Here's how the part is built. I have some questions about the finished solid (model axes, mm). A direction names the side the tool comes from. Round coordinates to 2 decimals unless told otherwise and drop trailing zeros. Write each loop counter-clockwise with the first axis right and the second up, starting at its lowest first coordinate (ties: lowest second). Pieces come first, ordered by that corner, then holes. Notation, with made-up numbers: M 71,8 L 85,8 A32 ccw 85,37 Z; hole C 14,15 d11. An arc over 180 degrees is marked long. Use one line per item in the form item = value. Start each with the question number.
Q1. I want a section at C-C on y = -13. List the corners of the cut face in (x, z) for me, and give its area (3 significant figures).
Q2. I want a section at B-B on y = 17.5. List the corners of the cut face in (x, z) for me.
Q3. I need wall thicknesses on line 1 along X through (y, z) = (-31, 13.25); line 2 along X through (y, z) = (-0.5, 5); line 3 along X through (y, z) = (-28, 2.75). Which ranges of each line are inside material? Lowest first, please. Write a range as from..to.
Q4. I want a section at A-A on z = 7.5. List the corners of the cut face in (x, y) for me, and give its area (3 significant figures).
Q5. We'd pull the mould along X, two halves only. Please class faces 4 (the face through (-19.46, -48.22, 7.4)), 5 (the face through (19.076, -48.375, 7.395)), 6 (the face through (0, 31, 8)): +X half, -X half, draft (parallel to the pull), parting line (faces both ways), or undercut.
Q6. I want a section at D-D on x = 43.5. List the corners of the cut face in (y, z) for me, and give its area (3 significant figures).
Q7. For faces 1 (the face through (5, -46, 8)), 2 (the face through (-46.99, 0.05, 6.25)), 3 (the face through (11, 1, 15)), which set-ups out of +Z, -Z, +X, -X, +Y, -Y let a thin tool reach every point of the face, with its end or its side?
Q8. I'm going to push flat-ended pins straight in: pin 1 Ø5 at (y, z) = (-18, 9.5) entering from +X; pin 2 Ø6 at (x, z) = (40.5, 13) entering from -Y; pin 3 Ø7.5 at (y, z) = (-15, 8.5) entering from +X. Where does each tip first touch, or does it pass through?
```python
from build123d import *

# Parameters (mm, degrees)
SKETCH1_R              = 52
BOSS_EXTRUDE1_DEPTH    = 15
CUT_EXTRUDE1_DEPTH     = 15
CUT_EXTRUDE2_DEPTH     = 30
M3_TAPPED_HOLE1_REACH  = 119.239
M3_TAPPED_HOLE1_BORE_R = 1.25


with BuildPart() as part:
    # Sketch1 → Boss-Extrude1 (new body)
    with BuildSketch(Plane.XY):
        Circle(SKETCH1_R)
    extrude(amount=BOSS_EXTRUDE1_DEPTH)

    # Sketch2 → Cut-Extrude1 (cut)
    with BuildSketch(Plane.XY.offset(15)):
        with BuildLine():
            Line((32, 0), (32, -45))
            Line((32, -45), (42, -45))
            Line((42, -45), (42, 3.54e-07))
            ThreePointArc((42, 3.54e-07), (36.999999823, 5), (32, 0))
        make_face()
        with BuildLine():
            Line((-5, -39.999999646), (-5, -55))
            Line((-5, -55), (5, -55))
            Line((5, -55), (5, -40))
            ThreePointArc((5, -40), (1.77e-07, -35), (-5, -39.999999646))
        make_face()
        with BuildLine():
            Line((-32, -45), (-42, -45))
            Line((-42, -45), (-42, 3.54e-07))
            ThreePointArc((-42, 3.54e-07), (-36.999999823, 5), (-32, 0))
            Line((-32, 0), (-32, -45))
        make_face()
    extrude(amount=-CUT_EXTRUDE1_DEPTH, mode=Mode.SUBTRACT)

    # Sketch3 → Cut-Extrude2 (cut)
    with BuildSketch(Plane.XY.offset(15)):
        with BuildLine():
            Line((4, 27.000000608), (4, -40))
            Line((4, -40), (-4, -40))
            Line((-4, -40), (-4, 27))
            ThreePointArc((-4, 27), (-3.04e-07, 31), (4, 27.000000608))
        make_face()
    extrude(amount=-CUT_EXTRUDE2_DEPTH, mode=Mode.SUBTRACT)

    # M3 Tapped Hole1 bore → M3 Tapped Hole1 (cut, up to next)
    with BuildSketch(Plane.ZY.offset(52), mode=Mode.PRIVATE) as m3_tapped_hole1_sk1:
        with Locations((7.5, 4.2e-08)):
            Circle(M3_TAPPED_HOLE1_BORE_R)
    m3_tapped_hole1_tool1 = extrude(m3_tapped_hole1_sk1.sketch, amount=-M3_TAPPED_HOLE1_REACH, mode=Mode.PRIVATE) & part.part
    m3_tapped_hole1 = m3_tapped_hole1_tool1.solids().sort_by_distance((-52, 0, 7.5))[0]
    add(m3_tapped_hole1, mode=Mode.SUBTRACT)

    # Mirror1: M3 Tapped Hole1 across plane
    add(m3_tapped_hole1.mirror(Plane(origin=(0, 0, 0), x_dir=(0, 0, 1), z_dir=(1, 0, 0))), mode=Mode.SUBTRACT)


solid = part.part
```
Reported:
q1.outline = M -50.35,0 L -42,0 L -42,15 L -50.35,15 Z; M -32,0 L -4,0 L -4,15 L -32,15 Z; M 4,0 L 32,0 L 32,15 L 4,15 Z; M 42,0 L 50.35,0 L 50.35,15 L 42,15 Z
q1.area = 1,090 mm^2
q2.outline = M -48.97,0 L -4,0 L -4,15 L -48.97,15 Z; M 4,0 L 48.97,0 L 48.97,15 L 4,15 Z
q3.line_1 = -32..-4, 4..32
q3.line_2 = -52..-42, -32..-4, 4..32, 42..52
q3.line_3 = -43.82..-42, -32..-4, 4..32, 42..43.82
q4.outline = M -51.98,-1.25 A52 ccw -42,-30.66 L -42,-1.25 Z; M -51.98,1.25 L -41.84,1.25 A5 cw -32,0 L -32,-40.99 A52 ccw -5,-51.76 L -5,-40 A5 cw -4,-37 L -4,27 A4 cw 4,27 L 4,-37 A5 cw 5,-40 L 5,-51.76 A52 ccw 32,-40.99 L 32,0 A5 cw 41.84,1.25 L 51.98,1.25 A52 ccw Z; M 42,-30.66 A52 ccw 51.98,-1.25 L 42,-1.25 Z
q4.area = 6,960 mm^2
q5.face_4 = -X half
q5.face_5 = +X half
q5.face_6 = undercut
q6.outline = M -28.49,0 L 28.49,0 L 28.49,15 L -28.49,15 Z; hole C 0,7.5 d2.5
q6.area = 850 mm^2
q7.face_1 = +Z, -Z, -Y
q7.face_2 = -X
q7.face_3 = +Z, +X, -X, +Y, -Y
q8.pin_1 = 49.64
q8.pin_2 = -30.66
q8.pin_3 = 50.77
